Here's how the part is built. I have some questions about the finished solid (model axes, mm). Face numbers are marked on the shaded views. A direction names the side the tool comes from. Round coordinates to 2 decimals unless told otherwise and drop trailing zeros. Loops run counter-clockwise (first coordinate to the right, second up) from the corner with the lowest first, then second, coordinate; pieces in that order, holes last. Notation, with made-up numbers: M 9,-26 L 20,-26 A31 cw 20,10 Z; hole C -2,3 d3. An arc over 180 degrees is marked long. Write item = value, one per line. Start each with the question number.
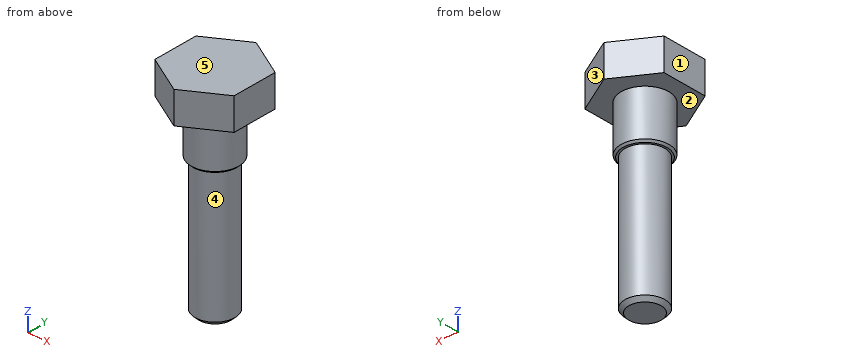
from build123d import *

# Parameters (mm, degrees)
F1_DEPTH = 12.7
F2_R     = 9.525
F3_DEPTH = 19.05
F4_R     = 7.9375
F5_DEPTH = 53.975
F6_SIZE  = 1.524
F7_SIZE  = 0.762


with BuildPart() as f1:
    # F0 (on Top) → F1 (new body)
    with BuildSketch(Plane.XY):
        Polygon((-15.875, 9.165436), (-15.875, -9.165436), (0, -18.330871), (15.875, -9.165436), (15.875, 9.165436), (0, 18.330871), align=None)
    extrude(amount=F1_DEPTH)

    # F2 (on face) → F3 (join)
    with BuildSketch(Plane(origin=(0, 0, 0), x_dir=(1, 0, 0), z_dir=(0, 0, -1))):
        Circle(F2_R)
    extrude(amount=F3_DEPTH)

    # F4 (on face) → F5 (join)
    with BuildSketch(Plane(origin=(0, 0, -19.05), x_dir=(1, 0, 0), z_dir=(0, 0, -1))):
        Circle(F4_R)
    extrude(amount=F5_DEPTH)

    # F6
    f6_edges = [f1.edges().sort_by_distance(p)[0] for p in [
        (-7.9375, 0, -73.025),
    ]]
    chamfer(f6_edges, length=F6_SIZE)

    # F7
    f7_edges = [f1.edges().sort_by_distance(p)[0] for p in [
        (-9.525, 0, -19.05),
    ]]
    chamfer(f7_edges, length=F7_SIZE)


solid = f1.part
Item 1: We'd pull the mould along Y, two halves only. Please class the marked faces 3, 4 and 5: released by +Y, released by -Y, zero draft, split by the parting line, or undercut.
Item 2: For the marked faces 1 and 2, which set-ups out of +Z, -Z, +X, -X, +Y, -Y let a thin tool reach every point of the face, with its end or its side?
Item 3: I want a section at D-D, the plane z = -58.5. List the corners of the cut face in (x, y) for me (1 decimal).
Item 4: Please list where these lines run through material, in increasing order: line 1 (Z direction, x = 1, y = 14); line 2 (Z direction, x = 0, y = 8); line 3 (X direction, y = 0, z = -33.5). Write a range as [from, to].
Item 5: I want a section at C-C, the plane x = 10.5. List the corners of the cut face in (y, z) for me, then the cut area to 3 significant figures.
Item 6: Will these pins go through, and if not, where does the flat tip stop? pin 1 Ø3 at (y, z) = (11, -1) entering from +X; pin 2 Ø5 at (x, z) = (-3.5, -50) entering from -Y; pin 3 Ø1.5 at (x, z) = (-6.5, -58.5) entering from +Y.
Item 7: I want a section at B-B, the plane z = -5. List the corners of the cut face in (x, y) for me (3 decimals).
Worked out:
q1.face_3 = released by +Y
q1.face_4 = split by the parting line
q1.face_5 = zero draft
q2.face_1 = +Z, -Z, -X, +Y, -Y
q2.face_2 = -Z
q3.outline = C 0,0 d15.9
q4.line_1 = [0, 12.7]
q4.line_2 = [-19.05, 12.7]
q4.line_3 = [-7.94, 7.94]
q5.outline = M -12.27,0 L 12.27,0 L 12.27,12.7 L -12.27,12.7 Z
q5.area = 312 mm2
q6.pin_1 = 14.63
q6.pin_2 = -7.87
q6.pin_3 = 5.47
q7.outline = C 0,0 d19.05
